```python
from build123d import *

# Parameters (mm, degrees)
EXTRUDE_1_DEPTH          = 5
EXTRUDE_2_DEPTH          = 5
CUT_EXTRUDE_1_DEPTH      = 5
CUT_EXTRUDE_2_REACH      = 7
SKETCH_5_R               = 1.524999999
SKETCH_6_R               = 2.025
CUT_EXTRUDE_3_DEPTH      = 1
CUT_EXTRUDE_3_DEPTH_BACK = 6
CUT_EXTRUDE_4_DEPTH      = 6
FILLET_4_R               = 2
SKETCH_8_R               = 7.5
CUT_EXTRUDE_5_DEPTH      = 5
EXTRUDE_3_DEPTH          = 5
SKETCH_10_R              = 7.025
CUT_EXTRUDE_6_DEPTH      = 5
FILLET_5_R               = 3


with BuildPart() as part:
    # 草图1 → 凸台-拉伸1 (new body)
    with BuildSketch(Plane.XY):
        Polygon((0, 0), (-55, 0), (-55, -30), (30, -30), (30, 50), (0, 50), align=None)
    extrude(amount=EXTRUDE_1_DEPTH)

    # 草图2 → 凸台-拉伸2 (add)
    with BuildSketch(Plane.XY.offset(5)):
        Polygon((0, 40), (-45, 0), (0, 0), align=None)
    extrude(amount=-EXTRUDE_2_DEPTH)

    # 草图4 → 切除-拉伸1 (cut)
    with BuildSketch(Plane.XY.offset(5)):
        Polygon((0, 33.310225234), (0, 0), (-37.474003388, 0), align=None)
    extrude(amount=-CUT_EXTRUDE_1_DEPTH, mode=Mode.SUBTRACT)

    # 草图5 → 切除-拉伸2 (cut, up to next)
    with BuildSketch(Plane(origin=(0, 0, 0), x_dir=(-1, 0, 0), z_dir=(0, 0, -1)), mode=Mode.PRIVATE) as cut_extrude_2_sk1:
        with Locations((48, -4.2)):
            Circle(SKETCH_5_R)
    cut_extrude_2_tool1 = extrude(cut_extrude_2_sk1.sketch, amount=-CUT_EXTRUDE_2_REACH, mode=Mode.PRIVATE) & part.part
    add(cut_extrude_2_tool1.solids().sort_by_distance((-48, -4.2, 0))[0], mode=Mode.SUBTRACT)
    # 草图5 → 切除-拉伸2 (cut, up to next)
    with BuildSketch(Plane(origin=(0, 0, 0), x_dir=(-1, 0, 0), z_dir=(0, 0, -1)), mode=Mode.PRIVATE) as cut_extrude_2_sk2:
        with Locations((48, -25.8)):
            Circle(SKETCH_5_R)
    cut_extrude_2_tool2 = extrude(cut_extrude_2_sk2.sketch, amount=-CUT_EXTRUDE_2_REACH, mode=Mode.PRIVATE) & part.part
    add(cut_extrude_2_tool2.solids().sort_by_distance((-48, -25.8, 0))[0], mode=Mode.SUBTRACT)
    # 草图5 → 切除-拉伸2 (cut, up to next)
    with BuildSketch(Plane(origin=(0, 0, 0), x_dir=(-1, 0, 0), z_dir=(0, 0, -1)), mode=Mode.PRIVATE) as cut_extrude_2_sk3:
        with Locations((28, -4.2)):
            Circle(SKETCH_5_R)
    cut_extrude_2_tool3 = extrude(cut_extrude_2_sk3.sketch, amount=-CUT_EXTRUDE_2_REACH, mode=Mode.PRIVATE) & part.part
    add(cut_extrude_2_tool3.solids().sort_by_distance((-28, -4.2, 0))[0], mode=Mode.SUBTRACT)
    # 草图5 → 切除-拉伸2 (cut, up to next)
    with BuildSketch(Plane(origin=(0, 0, 0), x_dir=(-1, 0, 0), z_dir=(0, 0, -1)), mode=Mode.PRIVATE) as cut_extrude_2_sk4:
        with Locations((28, -25.8)):
            Circle(SKETCH_5_R)
    cut_extrude_2_tool4 = extrude(cut_extrude_2_sk4.sketch, amount=-CUT_EXTRUDE_2_REACH, mode=Mode.PRIVATE) & part.part
    add(cut_extrude_2_tool4.solids().sort_by_distance((-28, -25.8, 0))[0], mode=Mode.SUBTRACT)

    # 草图6 → 切除-拉伸3 (cut, two sides)
    with BuildSketch(Plane(origin=(0, 0, 0), x_dir=(-1, 0, 0), z_dir=(0, 0, -1))) as cut_extrude_3_sk:
        with Locations((-6, 38)):
            Circle(SKETCH_6_R)
        with Locations((-24, 38)):
            Circle(SKETCH_6_R)
        with Locations((-24, 8)):
            Circle(SKETCH_6_R)
        with Locations((-6, 8)):
            Circle(SKETCH_6_R)
    extrude(amount=CUT_EXTRUDE_3_DEPTH, mode=Mode.SUBTRACT)
    extrude(cut_extrude_3_sk.sketch, amount=-CUT_EXTRUDE_3_DEPTH_BACK, mode=Mode.SUBTRACT)

    # 草图7 → 切除-拉伸4 (cut, through all)
    with BuildSketch(Plane(origin=(0, 0, 0), x_dir=(-1, 0, 0), z_dir=(0, 0, -1))):
        Polygon((12.750172416, -25), (-24, -8.295376175), (-24, -25), align=None)
        Polygon((20, -5), (-16.750172416, -5), (20, -21.704623825), align=None)
    extrude(amount=-CUT_EXTRUDE_4_DEPTH, mode=Mode.SUBTRACT)

    # 圆角4
    fillet_4_edges = [part.edges().sort_by_distance(p)[0] for p in [
        (16.750172416, -5, 2.5),
        (-20, -5, 2.5),
        (-20, -21.704623825, 2.5),
        (24, -8.295376175, 2.5),
        (-12.750172416, -25, 2.5),
        (24, -25, 2.5),
    ]]
    fillet(fillet_4_edges, radius=FILLET_4_R)

    # 草图8 → 切除-拉伸5 (cut)
    with BuildSketch(Plane(origin=(0, 0, 0), x_dir=(-1, 0, 0), z_dir=(0, 0, -1))):
        with Locations((-15, 23)):
            Circle(SKETCH_8_R)
    extrude(amount=-CUT_EXTRUDE_5_DEPTH, mode=Mode.SUBTRACT)

    # 草图9 → 凸台-拉伸3 (add)
    with BuildSketch(Plane.XY.offset(5)):
        Polygon((-55, 0), (0, 40), (0, 0), align=None)
    extrude(amount=-EXTRUDE_3_DEPTH)

    # 草图10 → 切除-拉伸6 (cut)
    with BuildSketch(Plane.XY.offset(5)):
        with Locations((-27, 8)):
            Circle(SKETCH_10_R)
        with Locations((-10, 20)):
            Circle(SKETCH_10_R)
    extrude(amount=-CUT_EXTRUDE_6_DEPTH, mode=Mode.SUBTRACT)

    # 圆角5
    fillet_5_edges = [part.edges().sort_by_distance(p)[0] for p in [
        (0, 50, 2.5),
        (30, 50, 2.5),
        (30, -30, 2.5),
        (-55, -30, 2.5),
        (-55, 0, 2.5),
        (0, 40, 2.5),
    ]]
    fillet(fillet_5_edges, radius=FILLET_5_R)


solid = part.part
```
Work out the finished part from the listing and answer in its coordinate system (mm). A direction names the side the tool comes from. Coordinates: 2 decimals unless noted, no trailing zeros. Write each loop counter-clockwise with the first axis right and the second up, starting at its lowest first coordinate (ties: lowest second). Pieces come first, ordered by that corner, then holes.
Q1. Determine the mould class of faces 1 (the face through (25.49, 39.37, 2.46)), 2 (the face through (-46.476, -4.133, 2.465)), 3 (the face through (-54.664, -0.149, 2.535)), 4 (the face through (-12, 2, 0)) for opening direction X: released by +X, released by -X, zero draft, split by the parting line, or undercut.
Q2. This flat-tipped pin is pushed along its axis until it touches: pin 1 Ø1.5 at (y, z) = (20, 4) entering from -X. Where does it stop, or does it pass through?
Q3. A cutting plane is placed at B-B, the plane y = 25.5. Give the vertices of the cut face in (x, z), then the cut area to 3 significant figures.
Q4. A cutting plane is placed at D-D, the plane z = 1.7. State how many separate pieces and enclosed holes the cut face has, then the cut area to 3 significant figures.
Q5. A cutting plane is placed at C-C, the plane x = 6. Give the vertices of the cut face in (y, z) (3 decimals), then the cut area to 3 significant figures.
Q6. Find the intervals of material crossed by line 1 (Y direction, x = -9, z = 0.8); line 2 (X direction, y = 36.5, z = 0.35); line 3 (X direction, y = -12, z = 4.3), in increasing order.
Q7. A cutting plane is placed at A-A, the plane x = -10. Give the vertices of the cut face in (y, z) (3 decimals), then the cut area to 3 significant figures.
Q8. Which of the six approach directions +Z, -Z, +X, -X, +Y, -Y give full straight-line access (tool end or side, diameter ignored) to faces 5 (the face through (15, 50, 2)), 6 (the face through (0, 44, 2)), 7 (the face through (-5.48, -23.39, 2.54))?
Findings below:
1. face 1: undercut
1. face 2: undercut
1. face 3: released by -X
1. face 4: zero draft
2. pin 1: stops at x = -28.53
3. outline: (-19.94, 0) - (-14.37, 0) - (-14.37, 5) - (-19.94, 5) - close; (-5.63, 0) - (7.93, 0) - (7.93, 5) - (-5.63, 5) - close; (22.07, 0) - (30, 0) - (30, 5) - (22.07, 5) - close
3. area: 135 mm2
4. separate pieces: 1
4. enclosed holes: 13
4. area: 3,990 mm2
5. outline: (-30, 0) - (-25, 0) - (-25, 5) - (-30, 5) - close; (-16.477, 0) - (-9.886, 0) - (-9.886, 5) - (-16.477, 5) - close; (-5, 0) - (5.975, 0) - (5.975, 5) - (-5, 5) - close; (10.025, 0) - (35.975, 0) - (35.975, 5) - (10.025, 5) - close; (40.025, 0) - (50, 0) - (50, 5) - (40.025, 5) - close
5. area: 292 mm2
6. line 1: y = -30 to -16.7, -5 to 13.05, 26.95 to 33.45
6. line 2: x = -4.81 to 4.64, 7.36 to 22.64, 25.36 to 30
6. line 3: x = -55 to -20, 1.35 to 15.85, 24 to 30
7. outline: (-30, 0) - (-17.159, 0) - (-17.159, 5) - (-30, 5) - close; (-5, 0) - (12.975, 0) - (12.975, 5) - (-5, 5) - close; (27.025, 0) - (32.727, 0) - (32.727, 5) - (27.025, 5) - close
7. area: 183 mm2
8. face 5: +Z, -Z, +X, -X, +Y
8. face 6: +Z, -Z, -X, +Y
8. face 7: +Z, -Z
